```python
from build123d import *

# Parameters (mm, degrees)
BOSS_EXTRUDE1_DEPTH = 19.05
SKETCH3_R           = 12.7
BOSS_EXTRUDE2_DEPTH = 25.4


with BuildPart() as part:
    # Sketch2 → Boss-Extrude1 (new body)
    with BuildSketch(Plane.XY):
        with BuildLine():
            Line((-14.199031657, 12.7), (14.199031657, 12.7))
            ThreePointArc((14.199031657, 12.7), (19.05, 0), (14.199031657, -12.7))
            Line((14.199031657, -12.7), (-14.199031657, -12.7))
            ThreePointArc((-14.199031657, -12.7), (-19.05, 0), (-14.199031657, 12.7))
        make_face()
    extrude(amount=BOSS_EXTRUDE1_DEPTH)

    # Sketch3 → Boss-Extrude2 (add)
    with BuildSketch(Plane.XY.offset(19.05)):
        Circle(SKETCH3_R)
    extrude(amount=BOSS_EXTRUDE2_DEPTH)


solid = part.part
```
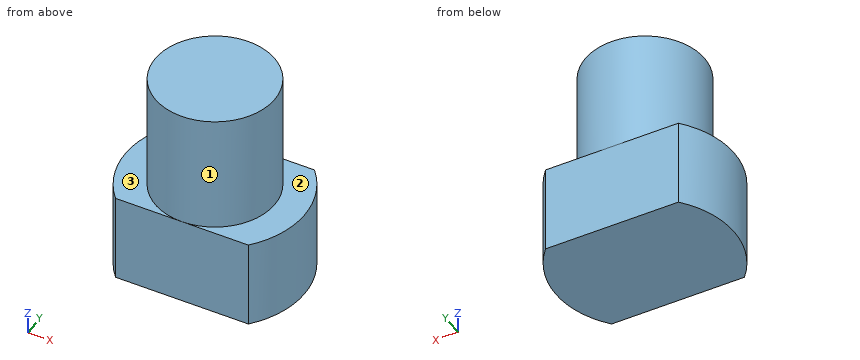
CAD build for the part. Positions are in the model's coordinates, mm. Face numbers are marked on the shaded views. A direction names the side the tool comes from. Round coordinates to 2 decimals unless told otherwise and drop trailing zeros. Write each loop counter-clockwise with the first axis right and the second up, starting at its lowest first coordinate (ties: lowest second). Pieces come first, ordered by that corner, then holes. Notation, with made-up numbers: (31, -12.5) -> (37, -12.5) arc R13 cw to (37, 5.5) -> close; hole circle Ø6 at (-3, 25). An arc over 180 degrees is marked (long way). Answer in a Markdown table with one row per item. Add a question column.
Item 1: Saw through at C-C, the plane z = 36. Write the cut outline in (x, y).
Item 2: Drill centre lines: line 1 (Z direction, x = 13, y = -4); line 2 (X direction, y = 0.5, z = 20); line 3 (X direction, y = 7, z = 23). Where is each one in solid material? Low to high. Write a range as from..to.
Item 3: Saw through at A-A, the plane y = 0. Write the cut outline in (x, z).
Item 4: Saw through at D-D, the plane z = 5. Write the cut outline in (x, y), then the cut area to 3 significant figures.
Item 5: Saw through at B-B, the plane x = 4.5. Write the cut outline in (y, z).
Item 6: Drop flat-ended pins along their axis: pin 1 Ø3 at (x, y) = (14.5, -6.5) entering from +Z; pin 2 Ø2 at (y, z) = (-1.5, 27.5) entering from +X; pin 3 Ø4 at (y, z) = (-1.5, 16) entering from +X. Give the stop position or say it passes through.
Item 7: Which spindle directions (+Z, -Z, +X, -X, +Y, -Y) get a long thin tool onto all of the face, cutting with end or side? Do the marked faces 1, 2 and 3. Say none if no direction does.
Findings below:
| question | item | result |
|---|---|---|
| 1 | outline | circle Ø25.4 at (0, 0) |
| 2 | line 1 | z = 0..19.05 |
| 2 | line 2 | x = -12.69..12.69 |
| 2 | line 3 | x = -10.6..10.6 |
| 3 | outline | (-19.05, 0) -> (19.05, 0) -> (19.05, 19.05) -> (12.7, 19.05) -> (12.7, 44.45) -> (-12.7, 44.45) -> (-12.7, 19.05) -> (-19.05, 19.05) -> close |
| 4 | outline | (-14.2, -12.7) -> (14.2, -12.7) arc R19.05 ccw to (14.2, 12.7) -> (-14.2, 12.7) arc R19.05 ccw to start |
| 4 | area | 890 mm^2 |
| 5 | outline | (-12.7, 0) -> (12.7, 0) -> (12.7, 19.05) -> (11.88, 19.05) -> (11.88, 44.45) -> (-11.88, 44.45) -> (-11.88, 19.05) -> (-12.7, 19.05) -> close |
| 6 | pin 1 | stops at z = 19.05 |
| 6 | pin 2 | stops at x = 12.69 |
| 6 | pin 3 | stops at x = 19.05 |
| 7 | face 1 | +Z |
| 7 | face 2 | +Z, +X |
| 7 | face 3 | +Z, -X |
